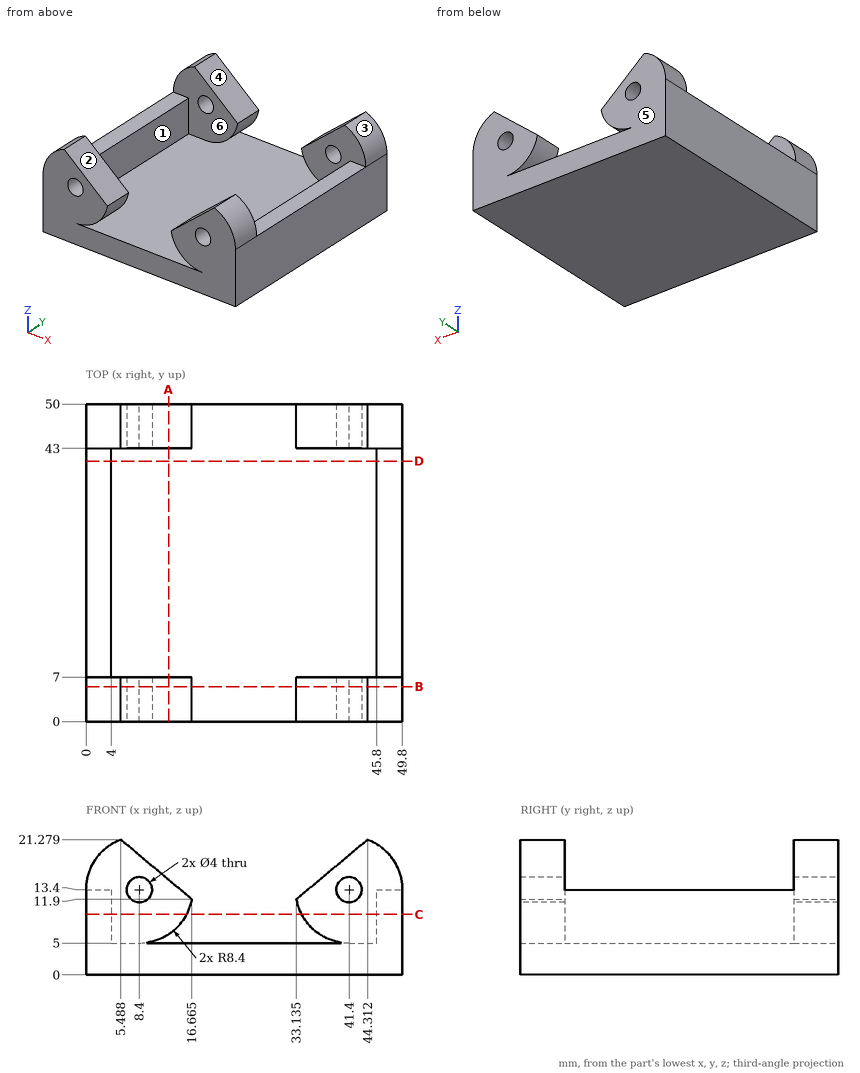
Part print with two shaded views. Sizes in mm from the minimum x, y, z corner. A direction names the side the tool comes from. Coordinates: 2 decimals unless noted, no trailing zeros. Order: outer loops, then holes, each group sorted by start corner. A loop starts at its lowest first (then second) coordinate and runs counter-clockwise, first axis right, second up. Notation, with made-up numbers: M 68.25,47.5 L 80.25,47.5 A8 cw 80.25,51.5 Z; hole C 74,53.5 d11. An arc over 180 degrees is marked long. Use a Markdown table: item, result.
(1) Flat gauge pins, fed straight in: pin 1 (3 mm diameter, centred on x = 6.5, y = 37, fed in from +Z); pin 2 (4.5 mm diameter, centred on x = 47, y = 31, fed in from +Z); pin 3 (2 mm diameter, centred on x = 14, y = 6.5, fed in from +Z) (1 decimal). Where does each tip first touch, or does it go through?
A:
| item | result |
|---|---|
| pin 1 | stops at z = 5 |
| pin 2 | stops at z = 13.4 |
| pin 3 | stops at z = 15 |
(2) Probe L1, parallel to Y at x = 11, z = 12.5; L2, parallel to X at y = 47.75, z = 13.4 (1 decimal); L3, parallel to X at y = 27, z = 6.75. List the from-to ranges inside material, lowest first.
A:
| item | result |
|---|---|
| L1 | y = 0 to 7, 43 to 50 |
| L2 | x = 0 to 6.4, 10.4 to 14.9, 34.9 to 39.4, 43.4 to 49.8 |
| L3 | x = 0 to 4, 45.8 to 49.8 |
(3) Cut at A-A on x = 13. Write the cut outline in (y, z) (1 decimal).
A:
| item | result |
|---|---|
| outline | M 0,0 L 50,0 L 50,5 L 0,5 Z; M 0,6.4 L 7,6.4 L 7,15 L 0,15 Z; M 43,6.4 L 50,6.4 L 50,15 L 43,15 Z |
(4) Tool access for the marked faces 1, 2 and 3: list every direction of +Z, -Z, +X, -X, +Y, -Y with a clear straight run to the whole face (end or side of a thin tool).
A:
| item | result |
|---|---|
| face 1 | +Z |
| face 2 | +Z, +Y, -Y |
| face 3 | +Z, +X, +Y, -Y |
(5) Pull direction Y, two halves, no side cores. Call the marked faces 4, 5 and 6: released by +Y, released by -Y, zero draft, split by the parting line, or undercut.
A:
| item | result |
|---|---|
| face 4 | zero draft |
| face 5 | released by +Y |
| face 6 | undercut |
(6) Cut at C-C on z = 9.5. Write the cut outline in (x, y).
A:
| item | result |
|---|---|
| outline | M 0,0 L 15.84,0 L 15.84,7 L 4,7 L 4,43 L 15.84,43 L 15.84,50 L 0,50 Z; M 33.96,0 L 49.8,0 L 49.8,50 L 33.96,50 L 33.96,43 L 45.8,43 L 45.8,7 L 33.96,7 Z |
(7) Cut at B-B on y = 5.5. Write the cut outline in (x, z) (1 decimal), then the cut area to 3 significant figures.
A:
| item | result |
|---|---|
| outline | M 0,0 L 49.8,0 L 49.8,13.4 A8.4 ccw 44.3,21.3 L 33.1,11.9 A8.4 ccw 41.4,5 L 8.4,5 A8.4 ccw 16.7,11.9 L 5.5,21.3 A8.4 ccw 0,13.4 Z; hole C 8.4,13.4 d4; hole C 41.4,13.4 d4 |
| area | 610 mm^2 |
(8) Cut at D-D on y = 41. Write the cut outline in (x, z), then the cut area to 3 significant figures.
A:
| item | result |
|---|---|
| outline | M 0,0 L 49.8,0 L 49.8,13.4 L 45.8,13.4 L 45.8,5 L 4,5 L 4,13.4 L 0,13.4 Z |
| area | 316 mm^2 |
